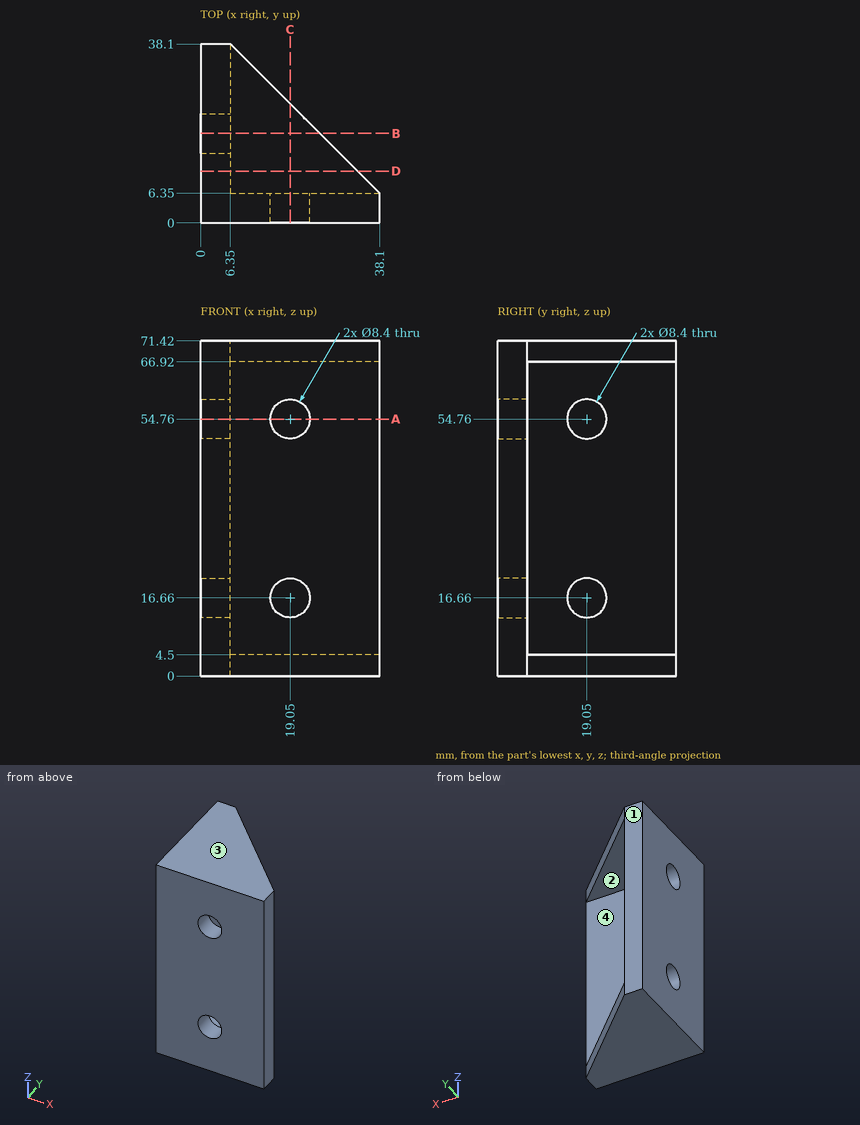
Verification items for this drawing (mm, ordinates from the low corner). Coordinates: 2 decimals unless noted, no trailing zeros. Loops run counter-clockwise (first coordinate to the right, second up) from the corner with the lowest first, then second, coordinate; pieces in that order, holes last.
Item 1: Thickness scan on line 1 (Z direction, x = 4, y = 19); line 2 (Z direction, x = 34, y = 9); line 3 (Y direction, x = 5, z = 54.76). Record the ranges inside material, lowest first.
Item 2: Sectioned sample at B-B, the plane y = 19.05. Record the boundary of the cut face in (x, z), then the cut area to 3 significant figures.
Item 3: Go/stop test with flat-tipped pins: pin 1 Ø16 at (y, z) = (15.5, 27.5) entering from +X; pin 2 Ø8 at (x, z) = (12, 33) entering from +Y; pin 3 Ø7.5 at (y, z) = (19.05, 54.76) entering from -X. Record where each tip stops, or that it passes through.
Item 4: Sectioned sample at A-A, the plane z = 54.76. Record the boundary of the cut face in (x, y), then the cut area to 3 significant figures.
Item 5: Sectioned sample at D-D, the plane y = 11. Record the boundary of the cut face in (x, z).
Item 6: Release check for a two-part mould opening along Z. For the marked faces 1, 2, 3 and 4 record: released by +Z, released by -Z, zero draft, split by the parting line, or undercut.
Check result:
1. line 1: z = 0 to 12.46, 20.86 to 50.56, 58.96 to 71.42
1. line 2: z = 0 to 4.5, 66.92 to 71.42
1. line 3: y = 0 to 14.85, 23.25 to 38.1
2. outline: (0, 0) - (25.4, 0) - (25.4, 4.5) - (6.35, 4.5) - (6.35, 12.46) - (0, 12.46) - close; (0, 20.86) - (6.35, 20.86) - (6.35, 50.56) - (0, 50.56) - close; (0, 58.96) - (6.35, 58.96) - (6.35, 66.92) - (25.4, 66.92) - (25.4, 71.42) - (0, 71.42) - close
2. area: 518 mm2
3. pin 1: stops at x = 6.35
3. pin 2: stops at y = 6.35
3. pin 3: passes through
4. outline: (0, 0) - (14.85, 0) - (14.85, 6.35) - (6.35, 6.35) - (6.35, 14.85) - (0, 14.85) - close; (0, 23.25) - (6.35, 23.25) - (6.35, 38.1) - (0, 38.1) - close; (23.25, 0) - (38.1, 0) - (38.1, 6.35) - (23.25, 6.35) - close
4. area: 337 mm2
5. outline: (0, 0) - (33.45, 0) - (33.45, 4.5) - (6.35, 4.5) - (6.35, 66.92) - (33.45, 66.92) - (33.45, 71.42) - (0, 71.42) - close
6. face 1: zero draft
6. face 2: undercut
6. face 3: released by +Z
6. face 4: undercut
